from build123d import *

# Parameters (mm, degrees)
F1_DEPTH  = 75
F3_R      = 3.442956
F4_DEPTH  = 49.9
F5_R      = 17.5
F6_DEPTH  = 1
F6_FACE_R = 17.5
F2_R      = 34.054107
F8_W      = 70
F8_H      = 2.474771
F8_H_2    = 23.374684
F9_DEPTH  = 35
F10_R     = 5
F11_R     = 16
F12_DEPTH = 10.3
F13_W     = 12
F13_H     = 7
F14_DEPTH = 3
F15_W     = 12
F15_H     = 7
F16_DEPTH = 3


with BuildPart() as f1:
    # F0 (on Front) → F1 (new body)
    with BuildSketch(Plane.XZ):
        Polygon((75, -17.5), (75, 17.5), (50, 17.5), (-50, 17.5), (-75, 17.5), (-75, -17.5), align=None)
        with BuildLine():
            Line((50, 17.5), (75, 17.5))
            ThreePointArc((75, 17.5), (62.5, 30), (50, 17.5))
        make_face()
        with BuildLine():
            Line((-75, 17.5), (-50, 17.5))
            ThreePointArc((-50, 17.5), (-62.5, 30), (-75, 17.5))
        make_face()
    extrude(amount=F1_DEPTH)

    # F3 (on face) → F4 (join)
    with BuildSketch(Plane.XY.offset(17.5)):
        with Locations((0, -37.356421)):
            Circle(F3_R)
    extrude(amount=F4_DEPTH)

    # F5 (on face) → F6 (join)
    with BuildSketch(Plane.XY.offset(67.4)):
        with Locations((0, -37.356421)):
            Circle(F5_R)
    extrude(amount=F6_DEPTH)

    # F6_face (on face) → F7 section 0
    with BuildSketch(Plane(origin=(0, -37.356421, 68.4), x_dir=(1, 0, 0), z_dir=(0, 0, 1))):
        Circle(F6_FACE_R)
    # F2 (on face) → F7 section 1
    with BuildSketch(Plane.XY.offset(17.5)):
        with Locations((0, -37.5)):
            Circle(F2_R)
    loft()

    # F8 (on face) → F9 (join)
    with BuildSketch(Plane.XY.offset(17.5)):
        with Locations((0, -1.237386)):
            Rectangle(F8_W, F8_H)
        with BuildLine():
            Line((-50, 0), (-35, 0))
            Line((-35, 0), (-35, 23.374684))
            ThreePointArc((-35, 23.374684), (-39.072516, 9.487857), (-50, 0))
        make_face()
        with Locations((0, 11.687342)):
            Rectangle(F8_W, F8_H_2)
        with BuildLine():
            Line((35, 23.374684), (35, 0))
            Line((35, 0), (50, 0))
            ThreePointArc((50, 0), (39.072516, 9.487857), (35, 23.374684))
        make_face()
    extrude(amount=-F9_DEPTH)

    # F10
    f10_edges = [f1.edges().sort_by_distance(p)[0] for p in [
        (35, 23.374684, 0),
        (-35, 23.374684, 0),
    ]]
    fillet(f10_edges, radius=F10_R)

    # F11 (on face) → F12 (join)
    with BuildSketch(Plane(origin=(0, 0, 0), x_dir=(-1, 0, 0), z_dir=(0, 1, 0))):
        with Locations((-55, 0)):
            Circle(F11_R)
        with Locations((55, 0)):
            Circle(F11_R)
    extrude(amount=F12_DEPTH)

    # F13 (on face) → F14 (cut)
    with BuildSketch(Plane.XY.offset(17.5)):
        with Locations((21, 12.874684)):
            Rectangle(F13_W, F13_H)
        with Locations((-21, 12.874684)):
            Rectangle(F13_W, F13_H)
    extrude(amount=-F14_DEPTH, mode=Mode.SUBTRACT)

    # F15 (on face) → F16 (cut)
    with BuildSketch(Plane(origin=(0, 0, -17.5), x_dir=(1, 0, 0), z_dir=(0, 0, -1))):
        with Locations((21, -14.107105)):
            Rectangle(F15_W, F15_H)
    extrude(amount=-F16_DEPTH, mode=Mode.SUBTRACT)


solid = f1.part
For this review, take the finished solid that the model builds, in its own axes (mm). A direction names the side the tool comes from. Round coordinates to 2 decimals unless told otherwise and drop trailing zeros. Write each loop counter-clockwise with the first axis right and the second up, starting at its lowest first coordinate (ties: lowest second). Pieces come first, ordered by that corner, then holes. Notation, with made-up numbers: (0, 48) -> (19, 48) arc R19 ccw to (19, 60) -> close; hole circle Ø5 at (-28, 59.25). An arc over 180 degrees is marked (long way). Use CSV: the item, a comma, the result in double quotes.
(1) To check wall thickness, follow L1, parallel to Z at x = 48, y = -53.5; L2, parallel to X at y = -36, z = 19; L3, parallel to Z at x = -22.5, y = 11.5. State the ranges of each line that lie inside material, in increasing order. Write a range as [from, to].
Computed values:
L1,"[-17.5, 17.5]"
L2,"[-74.91, -50.09], [-33.53, 33.53], [50.09, 74.91]"
L3,"[-17.5, 14.5]"
(2) Consider section B-B, the plane z = 2. Give the boundary of the cut face in (x, y).
Computed values:
outline,"(-75, -75) -> (75, -75) -> (75, 0) -> (70.87, 0) -> (70.87, 10.3) -> (39.13, 10.3) -> (39.13, 9.41) arc R25.71 cw to (35.34, 19.19) arc R5 ccw to (30.41, 23.37) -> (-30.41, 23.37) arc R5 ccw to (-35.34, 19.19) arc R25.71 cw to (-39.13, 9.41) -> (-39.13, 10.3) -> (-70.87, 10.3) -> (-70.87, 0) -> (-75, 0) -> close"
(3) Clearance check with flat-ended pins moving along their axes: P1, Ø12, axis at y = -50, z = 27.5, coming from the -X side; P2, Ø0.9, axis at y = 12.5, z = -16, coming from the -X side; P3, Ø0.9, axis at y = 11, z = 16, coming from the -X side. State where each tip first meets the part, or that it passes through.
Computed values:
P1,"x = -74.34"
P2,"x = -37.63"
P3,"x = -38.43"
(4) Draft analysis for pull direction X (two halves, no side actions). For faces 6 (the face through (-21, 16.375, 16)), 7 (the face through (15, 14, -16)), 8 (the face through (-33.607, 22.219, -0.245)), 9 (the face through (0, 23.375, 0)), state which applies: +X half, -X half, draft (parallel to the pull), parting line (faces both ways), or undercut.
Computed values:
face 6,"undercut"
face 7,"undercut"
face 8,"-X half"
face 9,"draft"
(5) Consider section C-C, the plane x = 43. Give the boundary of the cut face in (y, z), plus the area to 3 significant figures.
Computed values:
outline,"(-75, -17.5) -> (4.74, -17.5) -> (4.74, -10.58) -> (10.3, -10.58) -> (10.3, 10.58) -> (4.74, 10.58) -> (4.74, 17.5) -> (-75, 17.5) -> close"
area,"2,910 mm²"
(6) For faces 1 (the face through (55, 10.3, 0)), 2 (the face through (0, -37, 68.4)), 3 (the face through (27, 13, 16)), 4 (the face through (62.775, -36.975, 29.997)), 5 (the face through (21, 10.607, -16)), list the 3-axis set-ups (+Z, -Z, +X, -X, +Y, -Y) from which the entire face can be reached by the end or side of a thin tool; tool diameter is ignored.
Computed values:
face 1,"+Z, -Z, +X, +Y"
face 2,"+Z, +X, -X, +Y, -Y"
face 3,"+Z"
face 4,"+Z, +Y, -Y"
face 5,"-Z"
(7) Consider section A-A, the plane x = -55. Give the boundary of the cut face in (y, z), plus the area to 3 significant figures.
Computed values:
outline,"(-75, -17.5) -> (0, -17.5) -> (0, -16) -> (10.3, -16) -> (10.3, 16) -> (0, 16) -> (0, 27.5) -> (-75, 27.5) -> close"
area,"3,700 mm²"
